Autodesk Inventor part; units mm, degrees
ref_plane "YZ Plane" through (0, 0, 0) normal (1, 0, 0) x (0, 1, 0)
ref_plane "XZ Plane" through (0, 0, 0) normal (0, 1, 0) x (-1, 0, 0)
ref_plane "XY Plane" through (0, 0, 0) normal (0, 0, 1) x (1, 0, 0)
sketch "Sketch1" plane through (0, 0, 0) normal (0, 0, 1) x (1, 0, 0)
  line L0 (-70, 0) -> (-70, 70)
  line L1 (-70, 70) -> (-140, 70)
  line L2 (-140, 70) -> (-140, 53)
  line L3 (-140, 53) -> (-600, 53)
  line L4 (-600, 53) -> (-600, 70)
  line L5 (-600, 70) -> (-670, 70)
  line L6 (-670, 70) -> (-670, 0)
  line L7 (-670, 0) -> (-70, 0)
  point P0 (0, 0)
extrude "Extrusion1" add sketch "Sketch1" along normal blind 10
sketch "Sketch2" plane through (0, 0, 10) normal (0, 0, 1) x (1, 0, 0)
  line L0 (-70, 70) -> (-140, 70)
  line L1 (-70, 0) -> (-70, 70)
  line L2 (-600, 70) -> (-670, 70)
  line L3 (-670, 70) -> (-670, 0)
  point P0 (0, 0)
  point P1 (-105, 35)
  point P2 (-635, 35)
  dimension "d7" = 35
  dimension "d8" = 35
  dimension "d9" = 35
  dimension "d10" = 35
hole "Hole1" at (-105, 35, 10) at (-635, 35, 10) direction (0, 0, -1) diameter 18 end through all
sketch "Sketch3" plane through (0, 0, 10) normal (0, 0, 1) x (1, 0, 0)
  line L0 (-70, 70) -> (-140, 70)
  line L1 (-70, 0) -> (-70, 70)
  line L2 (-670, 0) -> (-70, 0)
  line L3 (-140, 70) -> (-140, 53)
  point P0 (0, 0)
  point P1 (-77, 63)
  point P2 (-77, 7)
  point P3 (-133, 63)
  point P4 (7, -7)
  dimension "d18" = 7
  dimension "d19" = 7
  dimension "d20" = 7
  dimension "d21" = 7
  dimension "d22" = 7
  dimension "d23" = 7
  dimension "d24" = 7
hole "Hole2" at (-77, 63, 10) at (-77, 7, 10) at (-133, 63, 10) at (7, -7, 10) direction (0, 0, -1) diameter 3 end through all
sketch "Sketch4" plane through (0, 0, 10) normal (0, 0, 1) x (1, 0, 0)
  line L0 (-670, 0) -> (-70, 0)
  line L1 (-70, 0) -> (-70, 70)
  point P0 (0, 0)
  point P1 (-133, 7)
  dimension "d32" = 7
  dimension "d33" = 63
hole "Hole3" at (-133, 7, 10) direction (0, 0, -1) diameter 3 end through all
sketch "Sketch5" plane through (0, 0, 10) normal (0, 0, 1) x (1, 0, 0)
  line L0 (-600, 70) -> (-670, 70)
  line L1 (-670, 70) -> (-670, 0)
  line L2 (-670, 0) -> (-70, 0)
  line L3 (-600, 53) -> (-600, 70)
  point P0 (0, 0)
  point P1 (-663, 63)
  point P2 (-663, 7)
  point P3 (-607, 63)
  point P4 (-607, 7)
  dimension "d41" = 7
  dimension "d42" = 7
  dimension "d43" = 7
  dimension "d44" = 7
  dimension "d45" = 7
  dimension "d46" = 7
  dimension "d47" = 7
  dimension "d48" = 63
hole "Hole4" at (-663, 63, 10) at (-663, 7, 10) at (-607, 63, 10) at (-607, 7, 10) direction (0, 0, -1) diameter 3 end through all
sketch "Sketch6" plane through (0, 0, 10) normal (0, 0, 1) x (1, 0, 0)
  line L0 (-140, 53) -> (-600, 53)
  point P0 (0, 0)
  point P1 (-581.6285, 35)
  point P2 (-142, 53)
  point P3 (-598, 53)
  dimension "d63" = 18
hole "Hole5" at (-581.6285, 35, 10) direction (0, 0, -1) diameter 4 end through all
pattern_linear "Rectangular Pattern1" count 6 spacing 85 along (1, 0, 0) of "Hole5"
sketch "Sketch10" plane through (-670, 0, 0) normal (-1, 0, 0) x (0, 0, 1)
  line L0 (10, 70) -> (10, 0)
  line L1 (0, 0) -> (10, 0)
  point P0 (5, 35)
  dimension "d100" = 5
  dimension "d101" = 35
hole "Hole9" at (-670, 35, 5) direction (1, 0, 0) diameter 2 depth 10 tip angle 118
properties part number "conveyor belt sideplank"
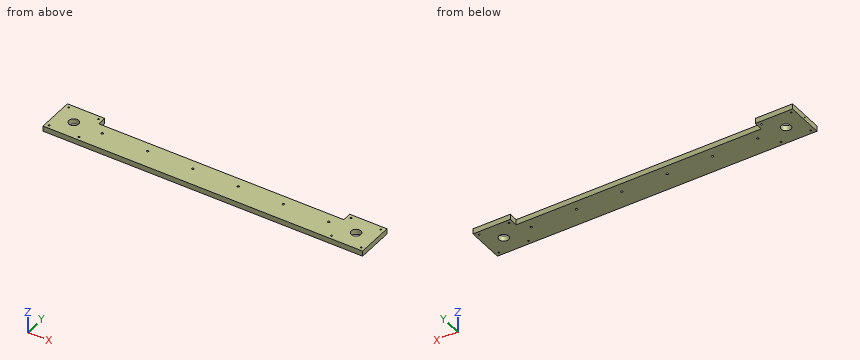
Read the model definition and answer for the solid it produces. Units are mm, in the model's axes. Give positions to 0.01 mm unless a question says otherwise; leave off trailing zeros. Order: outer loops, then holes, each group sorted by start corner. A loop starts at its lowest first (then second) coordinate and runs counter-clockwise, first axis right, second up.
(1) Straight lines are drawn through the part: L1, parallel to Y at x = -77, z = 4; L2, parallel to X at y = 63, z = 4.25; L3, parallel to X at y = 6, z = 5.75. For each, find the intervals that lie inside material, in ascending order.
(2) Given pin 1 (2 mm diameter, centred on x = -190, z = 3.5, fed in from +Y), flat-ended and moving along its own axis, determine where the tip first touches the part or whether it passes through.
(3) Find section A-A (x = -105). Give the vertices of the cut face in (y, z), plus the area to 3 significant figures.
(4) Find section C-C (x = -419.5). Give the vertices of the cut face in (y, z), plus the area to 3 significant figures.
(5) Find section B-B (z = 2.25). Give the number of separate pieces and of enclosed holes in the cut face, plus the area to 3 significant figures.
Result sheet:
1. L1: y = 0 to 5.5, 8.5 to 61.5, 64.5 to 70
1. L2: x = -670 to -664.5, -661.5 to -608.5, -605.5 to -600, -140 to -134.5, -131.5 to -78.5, -75.5 to -70
1. L3: x = -670 to -664.12, -661.88 to -608.12, -605.88 to -134.12, -131.88 to -78.12, -75.88 to -70
2. pin 1: stops at y = 53
3. outline: (0, 0) - (26, 0) - (26, 10) - (0, 10) - close; (44, 0) - (70, 0) - (70, 10) - (44, 10) - close
3. area: 520 mm2
4. outline: (0, 0) - (53, 0) - (53, 10) - (0, 10) - close
4. area: 530 mm2
5. separate pieces: 1
5. enclosed holes: 16
5. area: 33,500 mm2
